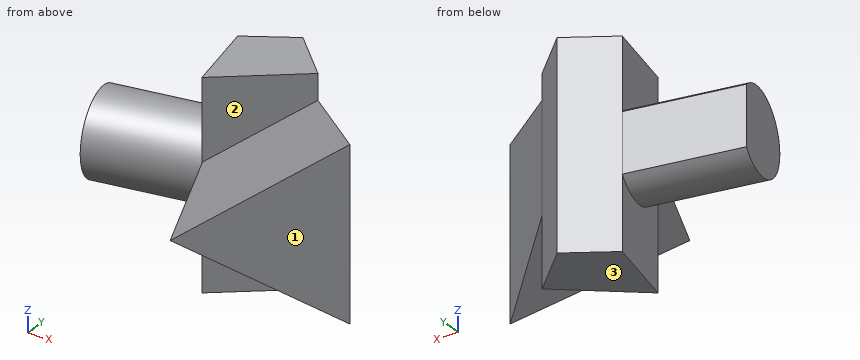
from build123d import *

# Parameters (mm, degrees)
F1_DEPTH      = 50.292
F1_DEPTH_BACK = 43.942
F3_DEPTH      = 51.054
F5_DEPTH      = 57.658
F5_TAPER      = -8


with BuildPart() as f1:
    # F0 (on Top) → F1 (new body, two sides)
    with BuildSketch(Plane.XY) as f1_sk:
        Polygon((-20.9554843605, 9.0488390997), (-14.5379882306, -24.1334326565), (19.8396630585, 3.1725820154), (0, 22.0344699919), align=None)
    extrude(amount=F1_DEPTH)
    extrude(f1_sk.sketch, amount=-F1_DEPTH_BACK)

    # F2 (on face) → F3 (join)
    with BuildSketch(Plane(origin=(-18.5129661664, -3.5804326358, 0), x_dir=(0.1898827546, -0.981806773, 0), z_dir=(-0.981806773, -0.1898827546, 0))):
        with BuildLine():
            ThreePointArc((-12.8632966108, -10.1028013332), (7.4441391901, -13.6647087453), (18.768443533, 3.5643151496))
            ThreePointArc((18.768443533, 3.5643151496), (7.4441391901, 20.7933390444), (-12.8632966108, 17.2314316323))
            Line((-12.8632966108, 17.2314316323), (-12.8632966108, -10.1028013332))
        make_face()
    extrude(amount=F3_DEPTH)

    # F4 (on face) → F5 (join)
    with BuildSketch(Plane(origin=(6.1297133792, -7.7171696999, 0), x_dir=(0.7830430091, 0.6219675601, 0), z_dir=(0.6219675601, -0.7830430091, 0))):
        Polygon((17.5085525567, -11.8831288274), (17.5085525567, 38.5248087551), (-26.1460019422, 13.3208399639), align=None)
    extrude(amount=F5_DEPTH, taper=F5_TAPER)


solid = f1.part
Design review of the part built by this model. Coordinates are the model's own, in mm. Face numbers are marked on the shaded views. Round coordinates to 2 decimals unless told otherwise and drop trailing zeros. Loops run counter-clockwise (first coordinate to the right, second up) from the corner with the lowest first, then second, coordinate; pieces in that order, holes last. Notation, with made-up numbers: M -24.75,23.5 L 32.25,23.5 A29 cw 32.25,57.5 Z; hole C -14.75,16 d6. An arc over 180 degrees is marked long. Answer as a JSON object with one key per item and string values.
Item 1: We need section A-A on z = -33.5. Give the boundary of the cut face in (x, y).
Answer sheet:
{"outline": "M -20.96,9.05 L -14.54,-24.13 L 19.84,3.17 L 0,22.03 Z"}
Item 2: Clearance check with flat-ended pins moving along their axes: P1, Ø5, axis at x = -35, z = -12.5, coming from the +Y side; P2, Ø12, axis at y = -4.5, z = -26, coming from the -X side; P3, Ø8, axis at x = -47.5, z = -15.5, coming from the +Y side. State where each tip first meets the part, or that it passes through.
Answer sheet:
{"P1": "stops at y = 6.47", "P2": "stops at x = -19.5", "P3": "stops at y = 2.27"}
Item 3: Wall thickness on L1, parallel to Z at x = -3, y = 5.5; L2, parallel to X at y = -14.5, z = 35; L3, parallel to X at y = -17.5, z = 41: over which ranges is each line inside the solid? List them lowest first. Write a range as from..to.
Answer sheet:
{"L1": "z = -43.94..50.29", "L2": "x = -16.4..-2.41, 20.88..38.44", "L3": "x = -15.82..-6.19, 32.99..41.59"}
Item 4: The part is to be moulded in two halves that separate along X. For the marked faces 1, 2 and 3, say which applies: pulls with the +X half, pulls with the -X half, needs draft (parallel to the pull), parting line crosses it, or undercut.
Answer sheet:
{"face 1": "pulls with the +X half", "face 2": "undercut", "face 3": "needs draft"}
